```python
from build123d import *

# Parameters (mm, degrees)
SKETCH_1_R      = 126.5
SKETCH_1_R_2    = 44.7
EXTRUDE_1_DEPTH = 3


with BuildPart() as part:
    # 草图1 → 凸台-拉伸1 (new body)
    with BuildSketch(Plane.XY):
        Circle(SKETCH_1_R)
        Circle(SKETCH_1_R_2, mode=Mode.SUBTRACT)
        with BuildLine():
            Line((-4, 118.232355978), (-4, 108.926580778))
            ThreePointArc((-4, 108.926580778), (-109, 0), (-4, -108.926580778))
            Line((-4, -108.926580778), (-4, -118.232355978))
            ThreePointArc((-4, -118.232355978), (-118.3, 0), (-4, 118.232355978))
        make_face(mode=Mode.SUBTRACT)
        with BuildLine():
            Line((4, 118.232355978), (4, 108.926580778))
            ThreePointArc((4, 108.926580778), (109, 0), (4, -108.926580778))
            Line((4, -108.926580778), (4, -118.232355978))
            ThreePointArc((4, -118.232355978), (118.3, 0), (4, 118.232355978))
        make_face(mode=Mode.SUBTRACT)
        with BuildLine():
            Line((4, -63.173491276), (4, -77.396705356))
            ThreePointArc((4, -77.396705356), (77.5, 0), (4, 77.396705356))
            Line((4, 77.396705356), (4, 63.173491276))
            ThreePointArc((4, 63.173491276), (63.3, 0), (4, -63.173491276))
        make_face(mode=Mode.SUBTRACT)
        with BuildLine():
            Line((-4, -63.173491276), (-4, -77.396705356))
            ThreePointArc((-4, -77.396705356), (-77.5, 0), (-4, 77.396705356))
            Line((-4, 77.396705356), (-4, 63.173491276))
            ThreePointArc((-4, 63.173491276), (-63.3, 0), (-4, -63.173491276))
        make_face(mode=Mode.SUBTRACT)
        with BuildLine():
            Line((-4, 99.919967974), (-4, 89.310469711))
            ThreePointArc((-4, 89.310469711), (-89.4, 0), (-4, -89.310469711))
            Line((-4, -89.310469711), (-4, -99.919967974))
            ThreePointArc((-4, -99.919967974), (-100, 0), (-4, 99.919967974))
        make_face(mode=Mode.SUBTRACT)
        with BuildLine():
            Line((4, 99.919967974), (4, 89.310469711))
            ThreePointArc((4, 89.310469711), (89.4, 0), (4, -89.310469711))
            Line((4, -89.310469711), (4, -99.919967974))
            ThreePointArc((4, -99.919967974), (100, 0), (4, 99.919967974))
        make_face(mode=Mode.SUBTRACT)
    extrude(amount=EXTRUDE_1_DEPTH)


solid = part.part
```
Check sheet for the modelled part. Datum: model origin and axes. Units: mm. A direction names the side the tool comes from. Give positions to 0.01 mm unless a question says otherwise; leave off trailing zeros. Loops run counter-clockwise (first coordinate to the right, second up) from the corner with the lowest first, then second, coordinate; pieces in that order, holes last. Notation, with made-up numbers: M -5.5,47 L 3.5,47 A25 cw 3.5,76 Z; hole C 72,17.5 d10. An arc over 180 degrees is marked long. Answer in a Markdown table with one row per item.
1) Cross-section at B-B (x = 0). Enter the section's corners in (y, z).
Solutions:
| item | result |
|---|---|
| outline | M -126.5,0 L -44.7,0 L -44.7,3 L -126.5,3 Z; M 44.7,0 L 126.5,0 L 126.5,3 L 44.7,3 Z |
2) Depth check by flat-ended pin: pin 1 (0.9 mm diameter, centred on y = -73.5, z = 2, fed in from -X); pin 2 (1.5 mm diameter, centred on y = -72, z = 2, fed in from +X); pin 3 (1 mm diameter, centred on x = 38, y = 50.5, fed in from -Z); pin 4 (5 mm diameter, centred on x = 62.5, y = 22.5, fed in from -Z) (3 decimals). Enter the tip coordinate at first touch or a pass-through.
Solutions:
| item | result |
|---|---|
| pin 1 | stops at x = -103.28 |
| pin 2 | stops at x = 104.53 |
| pin 3 | stops at z = 0 |
| pin 4 | passes through |
3) Cross-section at C-C (z = 2.45). Enter the section's corners in (x, y), plus the area to 3 significant figures.
Solutions:
| item | result |
|---|---|
| outline | C 0,0 d253; hole C 0,0 d89.4; hole M -4,-118.23 L -4,-108.93 A109 cw -4,108.93 L -4,118.23 A118.3 ccw Z; hole M -4,-99.92 L -4,-89.31 A89.4 cw -4,89.31 L -4,99.92 A100 ccw Z; hole M -4,-77.4 L -4,-63.17 A63.3 cw -4,63.17 L -4,77.4 A77.5 ccw Z; hole M 4,-118.23 A118.3 ccw 4,118.23 L 4,108.93 A109 cw 4,-108.93 Z; hole M 4,-99.92 A100 ccw 4,99.92 L 4,89.31 A89.4 cw 4,-89.31 Z; hole M 4,-77.4 A77.5 ccw 4,77.4 L 4,63.17 A63.3 cw 4,-63.17 Z |
| area | 25,300 mm^2 |
4) Mould release check, pull along Y, two halves, no side actions. Record for faces 1 (the face through (-99.977, -2.143, 1.479)), 2 (the face through (-16.468, 125.424, 1.479)), 3 (the face through (54, 2, 3)): released by +Y, released by -Y, zero draft, split by the parting line, or undercut.
Solutions:
| item | result |
|---|---|
| face 1 | undercut |
| face 2 | split by the parting line |
| face 3 | zero draft |
5) Thickness scan on line 1 (Y direction, x = 0, z = 1.9); line 2 (X direction, y = 91.5, z = 1.8); line 3 (Y direction, x = -66, z = 0.6). Record the ranges inside material, lowest first.
Solutions:
| item | result |
|---|---|
| line 1 | y = -126.5 to -44.7, 44.7 to 126.5 |
| line 2 | x = -87.35 to -74.98, -59.23 to -40.35, -4 to 4, 40.35 to 59.23, 74.98 to 87.35 |
| line 3 | y = -107.92 to -98.18, -86.75 to -75.13, -60.3 to -40.62, 40.62 to 60.3, 75.13 to 86.75, 98.18 to 107.92 |
6) Tool access check on faces 4 (the face through (108.975, 2.341, 1.479)), 5 (the face through (54, 2, 0)). Record the directions out of +Z, -Z, +X, -X, +Y, -Y that give a thin tool (end or side, any length) a straight path to the whole face; none if there is none.
Solutions:
| item | result |
|---|---|
| face 4 | +Z, -Z |
| face 5 | -Z, +X, -X, +Y, -Y |
7) Cross-section at A-A (y = 0). Count the separate pieces of the cut face and the enclosed holes in it, plus the area to 3 significant figures.
Solutions:
| item | result |
|---|---|
| separate pieces | 8 |
| enclosed holes | 0 |
| area | 286 mm^2 |
8) Cross-section at D-D (x = 48). Enter the section's corners in (y, z), plus the area to 3 significant figures.
Solutions:
| item | result |
|---|---|
| outline | M -117.04,0 L -108.12,0 L -108.12,3 L -117.04,3 Z; M -97.86,0 L -87.73,0 L -87.73,3 L -97.86,3 Z; M -75.42,0 L -60.85,0 L -60.85,3 L -75.42,3 Z; M -41.27,0 L 41.27,0 L 41.27,3 L -41.27,3 Z; M 60.85,0 L 75.42,0 L 75.42,3 L 60.85,3 Z; M 87.73,0 L 97.86,0 L 97.86,3 L 87.73,3 Z; M 108.12,0 L 117.04,0 L 117.04,3 L 108.12,3 Z |
| area | 449 mm^2 |
